Answer from the drawing. Dimensions are ordinates in mm from the lowest x, y and z of the part. Coordinates: 2 decimals unless noted, no trailing zeros. Order: outer loops, then holes, each group sorted by start corner. A loop starts at its lowest first (then second) coordinate and runs counter-clockwise, first axis right, second up. Notation, with made-up numbers: M 61,26 L 68,26 A9 ccw 68,38 Z; hole C 68,45.25 d10. An arc over 180 degrees is marked long. Use a Markdown table: item, result.
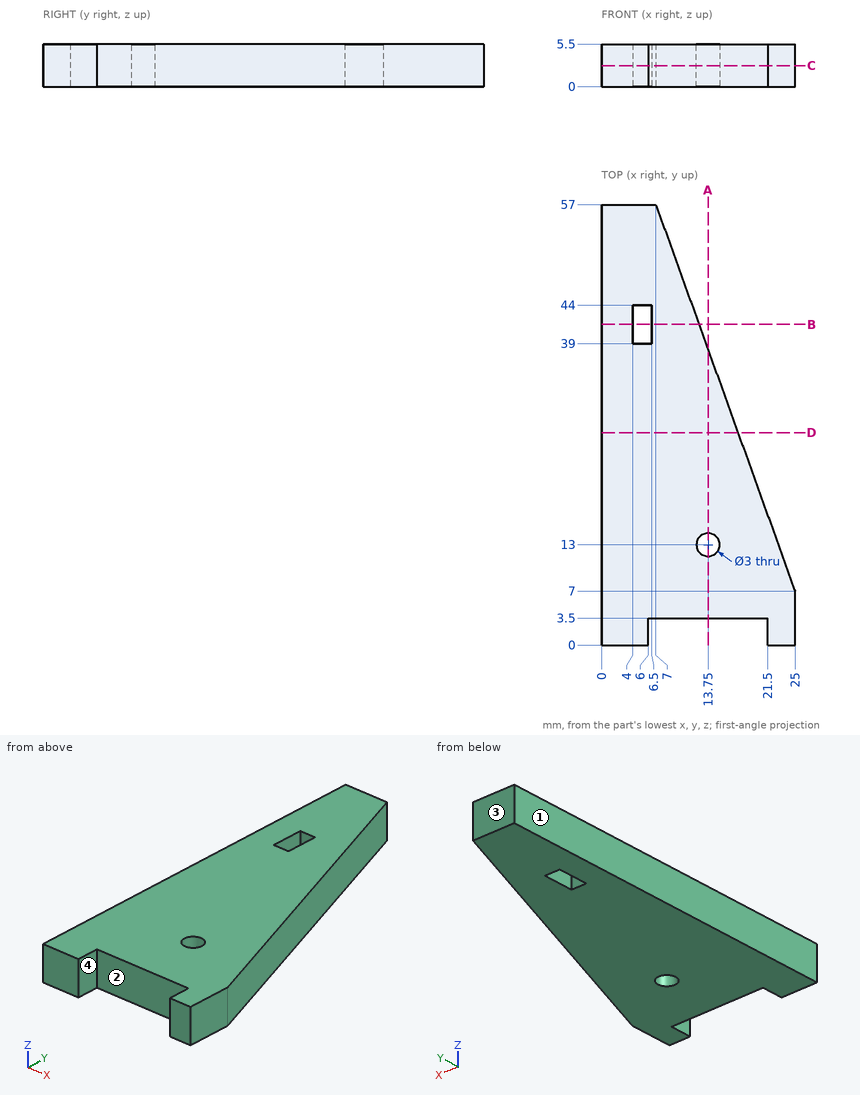
(1) Straight lines are drawn through the part: L1, parallel to X at y = 41.5, z = 0.7; L2, parallel to X at y = 24, z = 4.1; L3, parallel to X at y = 38.5, z = 1.8. For each, find the intervals that lie inside material, in ascending order.
Conclusion:
| item | result |
|---|---|
| L1 | 0 to 4, 6.5 to 12.58 |
| L2 | 0 to 18.88 |
| L3 | 0 to 13.66 |
(2) Given P1, Ø3, axis at x = 17.5, z = 3.5, coming from the -Y side; P2, Ø2, axis at x = 3.5, z = 2, coming from the -Y side, each flat-ended and moving along its own axis, determine where each tip first touches the part or whether it passes through.
Conclusion:
| item | result |
|---|---|
| P1 | y = 3.5 |
| P2 | y = 0 |
(3) Determine the mould class of the marked faces 1, 2, 3 and 4 for opening direction X: pulls with the +X half, pulls with the -X half, needs draft (parallel to the pull), parting line crosses it, or undercut.
Conclusion:
| item | result |
|---|---|
| face 1 | pulls with the -X half |
| face 2 | undercut |
| face 3 | needs draft |
| face 4 | undercut |
(4) A cutting plane is placed at A-A (x = 13.75). Determine the outline of the cut face in (y, z), then the cut area to 3 significant figures.
Conclusion:
| item | result |
|---|---|
| outline | M 3.5,0 L 11.5,0 L 11.5,5.5 L 3.5,5.5 Z; M 14.5,0 L 38.25,0 L 38.25,5.5 L 14.5,5.5 Z |
| area | 175 mm2 |
(5) A cutting plane is placed at C-C (z = 2.7). Determine the outline of the cut face in (x, y), then the cut area to 3 significant figures.
Conclusion:
| item | result |
|---|---|
| outline | M 0,0 L 6,0 L 6,3.5 L 21.5,3.5 L 21.5,0 L 25,0 L 25,7 L 7,57 L 0,57 Z; hole M 4,39 L 6.5,39 L 6.5,44 L 4,44 Z; hole C 13.75,13 d3 |
| area | 901 mm2 |
(6) A cutting plane is placed at D-D (y = 27.5). Determine the outline of the cut face in (x, z), then the cut area to 3 significant figures.
Conclusion:
| item | result |
|---|---|
| outline | M 0,0 L 17.62,0 L 17.62,5.5 L 0,5.5 Z |
| area | 96.9 mm2 |
(7) A cutting plane is placed at B-B (y = 41.5). Determine the outline of the cut face in (x, z).
Conclusion:
| item | result |
|---|---|
| outline | M 0,0 L 4,0 L 4,5.5 L 0,5.5 Z; M 6.5,0 L 12.58,0 L 12.58,5.5 L 6.5,5.5 Z |
